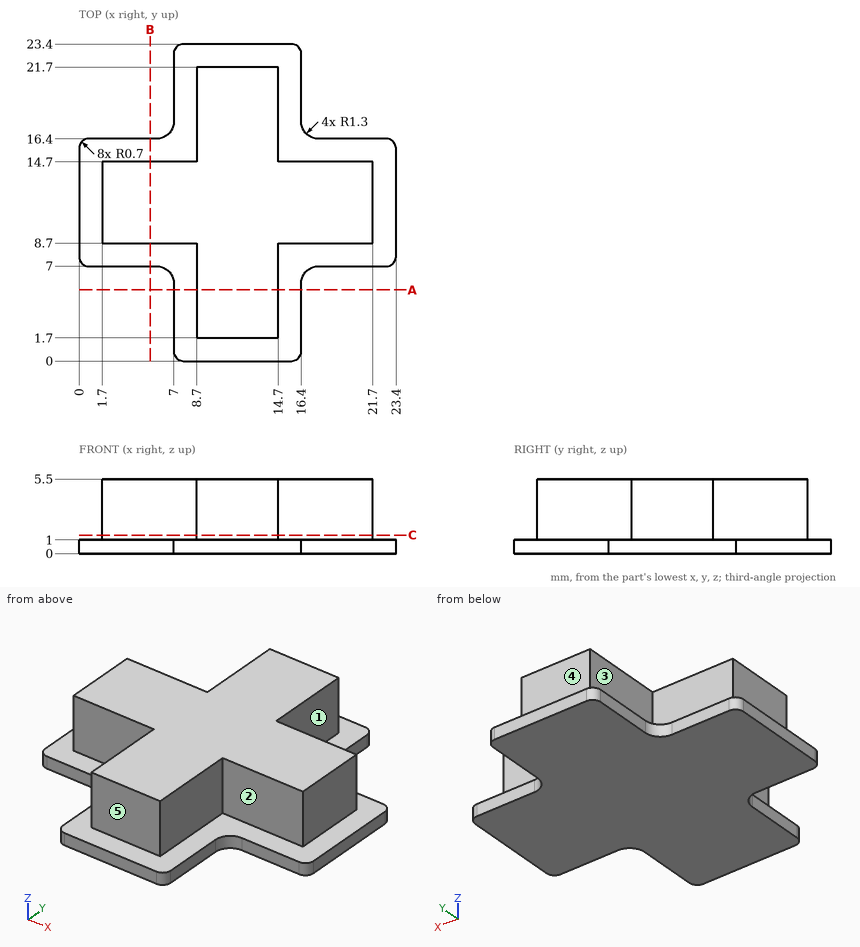
The drawing under review shows one solid part. Ordinate dimensions are in mm from its lowest x, y, z. A direction names the side the tool comes from. Give positions to 0.01 mm unless a question says otherwise; leave off trailing zeros. Order: outer loops, then holes, each group sorted by start corner. A loop starts at its lowest first (then second) coordinate and runs counter-clockwise, first axis right, second up. Notation, with made-up numbers: (-25, 4) -> (27, 4) arc R23 ccw to (27, 27) -> close; hole circle Ø8 at (62, 36). An arc over 180 degrees is marked (long way). Write item = value, one per line.
1) Insertion check: pin 1 (1.3 mm diameter, centred on x = 19.5, z = 3.5, fed in from +Y); pin 2 (0.5 mm diameter, centred on y = 20, z = 0.5, fed in from -X); pin 3 (1.1 mm diameter, centred on x = 21, z = 0.5, fed in from +Y). Each pin has a flat end and moves straight along its axis. Give the tip position at first contact, or say it passes through.
Findings:
pin_1 = 14.7
pin_2 = 7
pin_3 = 16.4
2) We need section A-A, the plane y = 5.25. Give the boundary of the cut face in (x, z), and give its area (3 significant figures).
Findings:
outline = (7, 0) -> (16.4, 0) -> (16.4, 1) -> (14.7, 1) -> (14.7, 5.5) -> (8.7, 5.5) -> (8.7, 1) -> (7, 1) -> close
area = 36.4 mm^2
3) For the marked faces 1, 2, 3, 4 and 5, list the 3-axis set-ups (+Z, -Z, +X, -X, +Y, -Y) from which the entire face can be reached by the end or side of a thin tool; tool diameter is ignored.
Findings:
face_1 = +Z, +X, +Y
face_2 = +Z, +X, -Y
face_3 = +Z, -X, +Y
face_4 = +Z, +X, -X, +Y
face_5 = +Z, +X, -X, -Y
4) To check wall thickness, follow L1, parallel to Y at x = 19.75, z = 0.5; L2, parallel to X at y = 6, z = 3.9. State the ranges of each line that lie inside material, in increasing order. Write a range as from..to.
Findings:
L1 = 7..16.4
L2 = 8.7..14.7
5) We need section C-C, the plane z = 1.35. Give the boundary of the cut face in (x, y).
Findings:
outline = (1.7, 8.7) -> (8.7, 8.7) -> (8.7, 1.7) -> (14.7, 1.7) -> (14.7, 8.7) -> (21.7, 8.7) -> (21.7, 14.7) -> (14.7, 14.7) -> (14.7, 21.7) -> (8.7, 21.7) -> (8.7, 14.7) -> (1.7, 14.7) -> close
